Part model, mm, in its own coordinate system. Face numbers are marked on the shaded views. A direction names the side the tool comes from. Round coordinates to 2 decimals unless told otherwise and drop trailing zeros. Write each loop counter-clockwise with the first axis right and the second up, starting at its lowest first coordinate (ties: lowest second). Pieces come first, ordered by that corner, then holes.
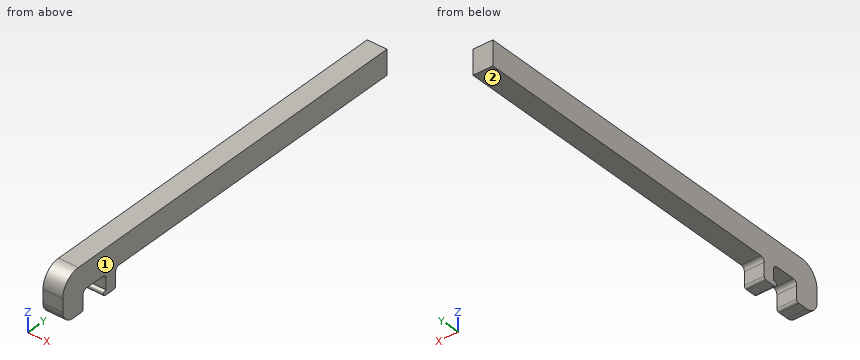
from build123d import *

# Parameters (mm, degrees)
F0_W     = 2
F0_H     = 2
F1_DEPTH = 1.5
F2_R     = 0.5
F5_DEPTH = 3
F6_W     = 70.54612
F6_H     = 32.912751
F7_DEPTH = 3.001


with BuildPart() as f1:
    # F0 (on Right) → F1 (new body, symmetric)
    with BuildSketch(Plane.YZ):
        with BuildLine():
            Line((-50, 0), (0, 0))
            Line((0, 0), (0, 4))
            Line((0, 4), (-57, 4))
            ThreePointArc((-57, 4), (-59.12132, 3.12132), (-60, 1))
            Line((-60, 1), (-60, 0))
            Line((-60, 0), (-56, 0))
            Line((-56, 0), (-52, 0))
            Line((-52, 0), (-50, 0))
        make_face()
        with Locations((-51, -1)):
            Rectangle(F0_W, F0_H)
        with BuildLine():
            Line((-50, -2.5), (-50, -2))
            Line((-50, -2), (-52, -2))
            Line((-52, -2), (-52, -3))
            Line((-52, -3), (-50.5, -3))
            ThreePointArc((-50.5, -3), (-50.146447, -2.853553), (-50, -2.5))
        make_face()
        with BuildLine():
            Line((-56, -2.5), (-56, 0))
            Line((-56, 0), (-60, 0))
            Line((-60, 0), (-60, -1))
            ThreePointArc((-60, -1), (-59.414214, -2.414214), (-58, -3))
            Line((-58, -3), (-56.5, -3))
            ThreePointArc((-56.5, -3), (-56.146447, -2.853553), (-56, -2.5))
        make_face()
        with BuildLine():
            Line((-52, -3), (-52, -2))
            ThreePointArc((-52, -2), (-52.5, -2.5), (-52, -3))
        make_face()
    extrude(amount=F1_DEPTH, both=True)

    # F2
    f2_edges = [f1.edges().sort_by_distance(p)[0] for p in [
        (0, -56, 0),
        (0, -52, 0),
        (0, -50, 0),
    ]]
    fillet(f2_edges, radius=F2_R)

    # F3: F1 across face


with BuildPart() as f1_1:
    add(f1.part)
    add(f1.part.mirror(Plane(origin=(0, 0, 2), x_dir=(-1, 0, 0), z_dir=(0, 1, 0))))

    # F4 (on face) → F5 (cut, through all)
    with BuildSketch(Plane.YZ.offset(1.5)):
        with BuildLine():
            Line((57, 4), (-57, 4))
            ThreePointArc((-57, 4), (-59.12132, 3.12132), (-60, 1))
            Line((-60, 1), (-60, -1))
            ThreePointArc((-60, -1), (-59.414214, -2.414214), (-58, -3))
            Line((-58, -3), (-56.5, -3))
            ThreePointArc((-56.5, -3), (-56.146447, -2.853553), (-56, -2.5))
            Line((-56, -2.5), (-56, -0.5))
            ThreePointArc((-56, -0.5), (-55.853553, -0.146447), (-55.5, 0))
            Line((-55.5, 0), (-52.5, 0))
            ThreePointArc((-52.5, 0), (-52.146447, -0.146447), (-52, -0.5))
            Line((-52, -0.5), (-52, -2))
            ThreePointArc((-52, -2), (-52.5, -2.5), (-52, -3))
            Line((-52, -3), (-50.5, -3))
            ThreePointArc((-50.5, -3), (-50.146447, -2.853553), (-50, -2.5))
            Line((-50, -2.5), (-50, -0.5))
            ThreePointArc((-50, -0.5), (-49.853553, -0.146447), (-49.5, 0))
            Line((-49.5, 0), (49.5, 0))
            Line((49.5, 0), (49.5, 0.125))
            Line((49.5, 0.125), (-49.5, 0.125))
            ThreePointArc((-49.5, 0.125), (-49.941942, -0.058058), (-50.125, -0.5))
            Line((-50.125, -0.5), (-50.125, -2.5))
            ThreePointArc((-50.125, -2.5), (-50.234835, -2.765165), (-50.5, -2.875))
            Line((-50.5, -2.875), (-52, -2.875))
            ThreePointArc((-52, -2.875), (-52.369599, -2.436587), (-51.875, -2.146447))
            Line((-51.875, -2.146447), (-51.875, -0.5))
            ThreePointArc((-51.875, -0.5), (-52.058058, -0.058058), (-52.5, 0.125))
            Line((-52.5, 0.125), (-55.5, 0.125))
            ThreePointArc((-55.5, 0.125), (-55.941942, -0.058058), (-56.125, -0.5))
            Line((-56.125, -0.5), (-56.125, -2.5))
            ThreePointArc((-56.125, -2.5), (-56.234835, -2.765165), (-56.5, -2.875))
            Line((-56.5, -2.875), (-58, -2.875))
            ThreePointArc((-58, -2.875), (-59.325825, -2.325825), (-59.875, -1))
            Line((-59.875, -1), (-59.875, 1))
            ThreePointArc((-59.875, 1), (-59.032932, 3.032932), (-57, 3.875))
            Line((-57, 3.875), (57, 3.875))
            Line((57, 3.875), (57, 4))
        make_face()
    extrude(amount=-F5_DEPTH, mode=Mode.SUBTRACT)

    # F6 (on face) → F7 (cut, through all)
    with BuildSketch(Plane.YZ.offset(1.5)):
        with Locations((35.27306, -3.023576)):
            Rectangle(F6_W, F6_H)
    extrude(amount=-F7_DEPTH, mode=Mode.SUBTRACT)


solid = f1_1.part
Q1. Drop flat-ended pins along their axis: P1, Ø0.9, axis at x = -0.5, y = -27, coming from the -Z side (3 decimals); P2, Ø1, axis at x = 0.5, z = -1.5, coming from the +Y side (3 decimals). Give the stop position or say it passes through.
Q2. Saw through at A-A, the plane x = 0.9. Write the cut outline in (y, z) (3 decimals).
Q3. Saw through at B-B, the plane y = -11. Write the cut outline in (x, z) (3 decimals), and give its area (4 significant figures).
Q4. Wall check: line 1 (Z direction, x = -0.1, y = -10.5) (3 decimals); line 2 (Y direction, x = 0.9, z = -1.75) (3 decimals); line 3 (Y direction, x = -0.9, z = -0.25) (3 decimals). Give the ranges that are in metal, low to high.
Q5. Tool access for the marked faces 1 and 2: list every direction of +Z, -Z, +X, -X, +Y, -Y with a clear straight run to the whole face (end or side of a thin tool).
Computed:
1. P1: stops at z = 0.125
1. P2: stops at y = -50.125
2. outline: (-59.875, -1) arc R1.875 ccw to (-58, -2.875) - (-56.5, -2.875) arc R0.375 ccw to (-56.125, -2.5) - (-56.125, -0.5) arc R0.625 cw to (-55.5, 0.125) - (-52.5, 0.125) arc R0.625 cw to (-51.875, -0.5) - (-51.875, -2.146) arc R0.375 ccw (long way) to (-52, -2.875) - (-50.5, -2.875) arc R0.375 ccw to (-50.125, -2.5) - (-50.125, -0.5) arc R0.625 cw to (-49.5, 0.125) - (0, 0.125) - (0, 3.875) - (-57, 3.875) arc R2.875 ccw to (-59.875, 1) - close
3. outline: (-1.5, 0.125) - (1.5, 0.125) - (1.5, 3.875) - (-1.5, 3.875) - close
3. area: 11.25 mm2
4. line 1: z = 0.125 to 3.875
4. line 2: y = -59.718 to -56.125, -51.875 to -50.125
4. line 3: y = -59.875 to -56.073, -51.927 to -50.073
5. face 1: +Z, -Z, +X, +Y, -Y
5. face 2: -Z, +X, -X, +Y
